```python
from build123d import *

# Parameters (mm, degrees)
SKETCH_W     = 46
SKETCH_H     = 10
PAD_DEPTH    = 2
SKETCH001_W  = 46
SKETCH001_H  = 2
PAD001_DEPTH = 46
PAD002_DEPTH = 2
SKETCH003_R  = 1.6
POCKET_DEPTH = 2.001


with BuildPart() as part:
    # Sketch → Pad (new body)
    with BuildSketch(Plane.XY):
        Rectangle(SKETCH_W, SKETCH_H)
    extrude(amount=PAD_DEPTH)

    # Sketch001 (on Face6 of Pad) → Pad001 (join)
    with BuildSketch(Plane.XY.offset(2)):
        with Locations((0, -4)):
            Rectangle(SKETCH001_W, SKETCH001_H)
    extrude(amount=PAD001_DEPTH)

    # Sketch002 (on Face8 of Pad001) → Pad002 (join)
    with BuildSketch(Plane.YZ.offset(23)):
        Polygon((-3, 48), (5, 2), (-3, 2), align=None)
    pad002 = extrude(amount=-PAD002_DEPTH)

    # Mirrored: Pad002 across YZ
    add(pad002.mirror(Plane.YZ))

    # Sketch003 (on Face5 of Mirrored) → Pocket (cut, through all)
    with BuildSketch(Plane.XY.offset(2)):
        with Locations((-12.5, 1)):
            Circle(SKETCH003_R)
        with Locations((12.5, 1)):
            Circle(SKETCH003_R)
    extrude(amount=-POCKET_DEPTH, mode=Mode.SUBTRACT)


solid = part.part
```
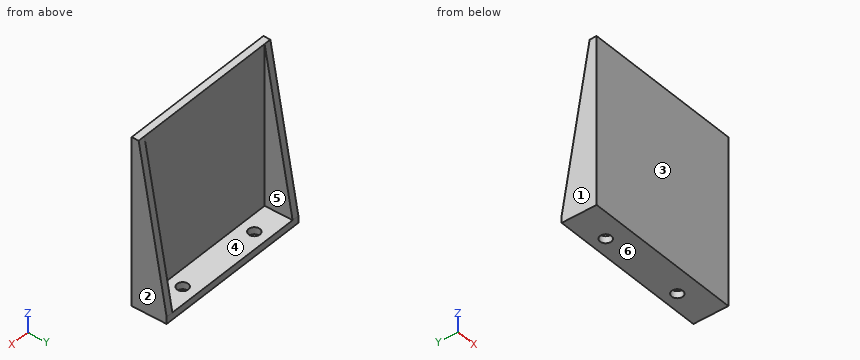
CAD build for the part. Positions are in the model's coordinates, mm. Face numbers are marked on the shaded views. A direction names the side the tool comes from. Round coordinates to 2 decimals unless told otherwise and drop trailing zeros. Loops run counter-clockwise (first coordinate to the right, second up) from the corner with the lowest first, then second, coordinate; pieces in that order, holes last. Notation, with made-up numbers: (44.25, 3.5) - (94.25, 3.5) arc R18 ccw to (94.25, 16.5) - close; hole circle Ø4 at (49, 50.5). An arc over 180 degrees is marked (long way). Return JSON: item names as keys, results as strings. Group by question number.
Q1. Flat gauge pins, fed straight in: pin 1 Ø8 at (x, z) = (9.5, 17) entering from +Y; pin 2 Ø1 at (x, y) = (11.5, 1) entering from +Z; pin 3 Ø2.5 at (x, y) = (8, 0.5) entering from +Z. Where does each tip first touch, or does it go through?
Q2. Band-saw the part on B-B on x = -12.5. Give the cut face in (y, z).
Q3. Band-saw the part on D-D on x = 4. Give the cut face in (y, z).
Q4. Drill centre lines: line 1 along Y through (x, z) = (-12.5, 0.5); line 2 along X through (y, z) = (-1, 8); line 3 along Y through (x, z) = (12, 1). Where is each one in solid material? Low to high. Write a range as [from, to].
Q5. Band-saw the part on C-C on z = 23. Give the cut face in (x, y), plus the area to 3 significant figures.
Q6. Tool access for the marked faces 5 and 6: list every direction of +Z, -Z, +X, -X, +Y, -Y with a clear straight run to the whole face (end or side of a thin tool).
Q7. Band-saw the part on A-A on y = 1. Give the cut face in (x, z), plus the area to 3 significant figures.
Q8. Two-plate mould, pull along X, no slides. Class the marked faces 1, 2, 3 and 4: +X half, -X half, draft (parallel to the pull), parting line (faces both ways), or undercut.
Solutions:
{
 "1": {"pin 1": "stops at y = -3", "pin 2": "passes through", "pin 3": "stops at z = 2"},
 "2": {"outline": "(-5, 0) - (-0.6, 0) - (-0.6, 2) - (-3, 2) - (-3, 48) - (-5, 48) - close; (2.6, 0) - (5, 0) - (5, 2) - (2.6, 2) - close"},
 "3": {"outline": "(-5, 0) - (5, 0) - (5, 2) - (-3, 2) - (-3, 48) - (-5, 48) - close"},
 "4": {"line 1": "y = [-5, -0.6], [2.6, 5]", "line 2": "x = [-23, -21], [21, 23]", "line 3": "y = [-5, -0.52], [2.52, 5]"},
 "5": {"outline": "(-23, -5) - (23, -5) - (23, 1.35) - (21, 1.35) - (21, -3) - (-21, -3) - (-21, 1.35) - (-23, 1.35) - close", "area": "109 mm^2"},
 "6": {"face 5": "+Z, +Y", "face 6": "-Z, +X, -X, +Y, -Y"},
 "7": {"outline": "(-23, 0) - (-14.1, 0) - (-14.1, 2) - (-21, 2) - (-21, 25) - (-23, 25) - close; (-10.9, 0) - (10.9, 0) - (10.9, 2) - (-10.9, 2) - close; (14.1, 0) - (23, 0) - (23, 25) - (21, 25) - (21, 2) - (14.1, 2) - close", "area": "171 mm^2"},
 "8": {"face 1": "-X half", "face 2": "+X half", "face 3": "draft", "face 4": "undercut"}
}
